Study the drawing (mm; zero at the part's minimum x, y, z) and answer. A direction names the side the tool comes from. Give positions to 0.01 mm unless a question says otherwise; leave off trailing zeros. Order: outer loops, then holes, each group sorted by start corner. A loop starts at its lowest first (then second) coordinate and runs counter-clockwise, first axis right, second up.
Item 1: Find the intervals of material crossed by line 1 along X through (y, z) = (1.85, 6); line 2 along Y through (x, z) = (32, 18); line 3 along Z through (x, y) = (24.5, 8.5), in increasing order.
Item 2: A cutting plane is placed at A-A (z = 26.5). Write down the section's boundary in (x, y).
Item 3: A cutting plane is placed at C-C (y = 3). Write down the section's boundary in (x, z), plus the area to 3 significant figures.
Item 4: A cutting plane is placed at B-B (x = 24.5). Write down the section's boundary in (y, z), plus the area to 3 significant figures.
Item 5: A cutting plane is placed at D-D (z = 39). Write down the section's boundary in (x, y), plus the area to 3 significant figures.
Item 6: Which of the six approach directions +Z, -Z, +X, -X, +Y, -Y give full straight-line access (tool end or side, diameter ignored) to the marked faces 4, 5, 6, 7 and 8?
Item 7: The mould has two halves that part along Y. Classify the marked faces 1, 2 and 3: +Y half, -Y half, draft (parallel to the pull), parting line (faces both ways), or undercut.
Item 8: Given pin 1 Ø5 at (y, z) = (28.5, 15) entering from +X; pin 2 Ø4 at (x, z) = (42.5, 38) entering from +Y; pin 3 Ø2.5 at (y, z) = (28.5, 15) entering from -X, each flat-ended and moving along its own axis, determine where each tip first touches the part or whether it passes through.
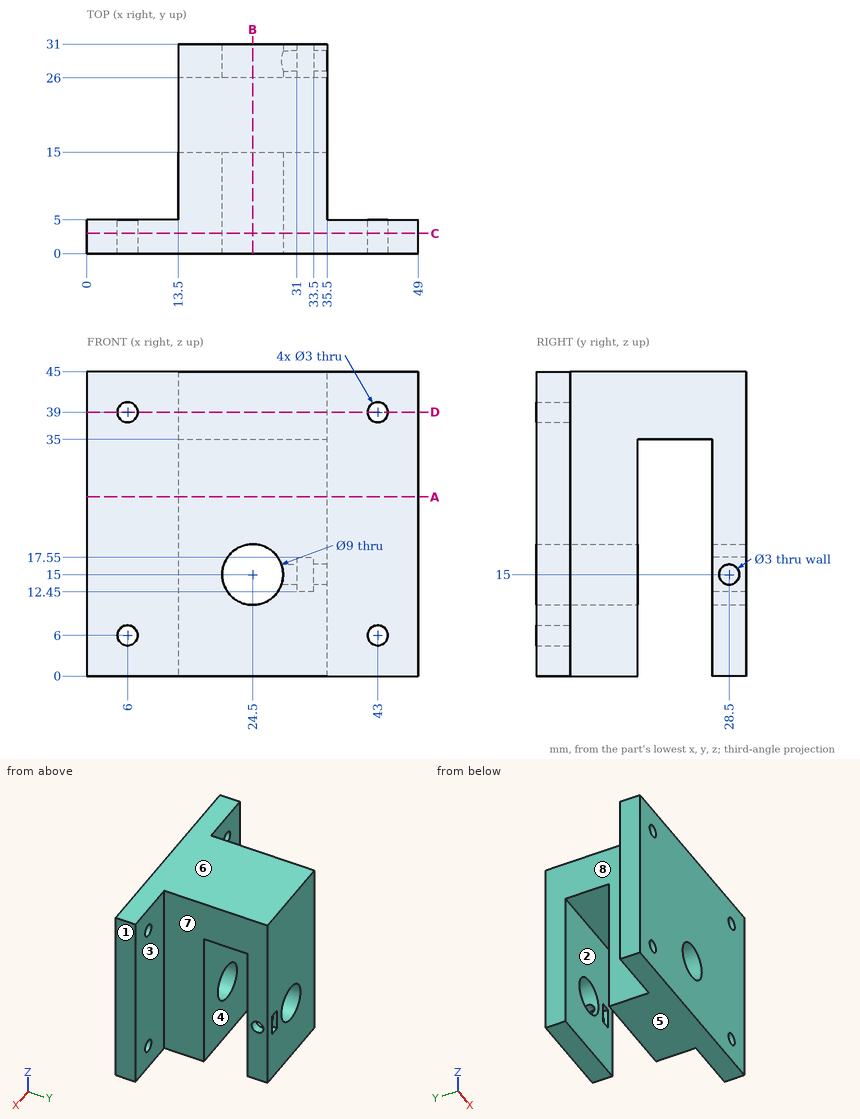
Response values:
1. line 1: x = 0 to 4.5, 7.5 to 41.5, 44.5 to 49
1. line 2: y = 0 to 15, 26 to 31
1. line 3: z = 0 to 10.5, 19.5 to 45
2. outline: (0, 0) - (49, 0) - (49, 5) - (35.5, 5) - (35.5, 15) - (13.5, 15) - (13.5, 5) - (0, 5) - close; (13.5, 26) - (35.5, 26) - (35.5, 31) - (13.5, 31) - close
3. outline: (0, 0) - (49, 0) - (49, 45) - (0, 45) - close; hole circle Ø3 at (6, 6); hole circle Ø3 at (6, 39); hole circle Ø9 at (24.5, 15); hole circle Ø3 at (43, 6); hole circle Ø3 at (43, 39)
3. area: 2,110 mm2
4. outline: (0, 0) - (15, 0) - (15, 10.5) - (0, 10.5) - close; (0, 19.5) - (15, 19.5) - (15, 35) - (26, 35) - (26, 19.5) - (31, 19.5) - (31, 45) - (0, 45) - close; (26, 0) - (31, 0) - (31, 10.5) - (26, 10.5) - close
4. area: 830 mm2
5. outline: (0, 0) - (4.5, 0) - (4.5, 5) - (0, 5) - close; (7.5, 0) - (41.5, 0) - (41.5, 5) - (35.5, 5) - (35.5, 31) - (13.5, 31) - (13.5, 5) - (7.5, 5) - close; (44.5, 0) - (49, 0) - (49, 5) - (44.5, 5) - close
5. area: 787 mm2
6. face 4: -Z, +X, -X
6. face 5: -Z, +X, -X, +Y, -Y
6. face 6: +Z, +X, -X, +Y, -Y
6. face 7: +Z, -Z, +X, +Y
6. face 8: +Z, -Z, -X, +Y
7. face 1: draft
7. face 2: undercut
7. face 3: +Y half
8. pin 1: stops at x = 35.5
8. pin 2: stops at y = 5
8. pin 3: stops at x = 13.5
